Geometry check sheet. Reference: the model listing, model coordinates, mm. A direction names the side the tool comes from. Coordinates: 2 decimals unless noted, no trailing zeros. Loops run counter-clockwise (first coordinate to the right, second up) from the corner with the lowest first, then second, coordinate; pieces in that order, holes last.
Autodesk Inventor part; units mm, degrees
ref_plane "YZ Plane" through (0, 0, 0) normal (1, 0, 0) x (0, 1, 0)
ref_plane "XZ Plane" through (0, 0, 0) normal (0, 1, 0) x (-1, 0, 0)
ref_plane "XY Plane" through (0, 0, 0) normal (0, 0, 1) x (1, 0, 0)
sketch "Sketch1" plane through (0, 0, 0) normal (1, 0, 0) x (0, 1, 0)
  line L0 (0, 0) -> (2400.3, 0)
  line L1 (2400.3, 0) -> (2400.3, -990.6)
  line L2 (2400.3, -990.6) -> (0, -990.6)
  line L3 (0, -990.6) -> (0, 0)
  dimension "d0" = 990.6
  dimension "d1" = 2400.3
extrude "Extrusion1" add sketch "Sketch1" along normal blind 127
sketch "Sketch2" plane through (127, 0, 0) normal (1, 0, 0) x (0, 0, -1)
  line L0 (0, 0) -> (990.6, 0)
  line L1 (927.1, 0) -> (63.5, 0)
  line L2 (63.5, 0) -> (63.5, 2082.8)
  line L3 (63.5, 2082.8) -> (927.1, 2082.8)
  line L4 (927.1, 2082.8) -> (927.1, 0)
  line L5 (990.6, 0) -> (990.6, 2400.3)
  point P0 (63.5, 0)
  point P1 (63.5, 0)
  dimension "d4" = 2082.8
  dimension "d6" = 63.5
  dimension "d7" = 863.6
extrude "Extrusion2" cut sketch "Sketch2" against normal up to surface (127 mm away)
properties part number "Wall_With_Door_For_Attic_Room" material "Wood (Southern Pine)"
1) Mould release check, pull along Z, two halves, no side actions. Record for faces 3 (the flat face through (63, 1217, -990.6)), 4 (the flat face through (64, 1056, -927.1)), 5 (the flat face through (64, 2082.8, -489)), 6 (the flat face through (63, 1183, 0)): +Z half, -Z half, draft (parallel to the pull), parting line (faces both ways), or undercut.
Data:
face 3: -Z half
face 4: undercut
face 5: undercut
face 6: +Z half
2) Section check C-C on z = -740. Record the cut outline in (x, y).
Data:
outline: (0, 2082.8) - (127, 2082.8) - (127, 2400.3) - (0, 2400.3) - close
3) Material ranges on probe 1 along Z at (x, y) = (20, 1375); probe 2 along Y at (x, z) = (117, -202.5), recorded low to high.
Data:
probe 1: z = -990.6 to -927.1, -63.5 to 0
probe 2: y = 2082.8 to 2400.3
4) Section check B-B on x = 40.5. Record the cut outline in (y, z).
Data:
outline: (0, -990.6) - (2400.3, -990.6) - (2400.3, 0) - (0, 0) - (0, -63.5) - (2082.8, -63.5) - (2082.8, -927.1) - (0, -927.1) - close
5) Access from +Z, -Z, +X, -X, +Y, -Y to the whole of each face (thin tool, end or side, straight path). Record for faces 1 (the flat face through (0, 2084, -493)), 2 (the flat face through (64, 1027, -63.5)).
Data:
face 1: +Z, -Z, -X, +Y, -Y
face 2: +X, -X, -Y
6) Section check A-A on y = 173. Record the cut outline in (x, z).
Data:
outline: (0, -990.6) - (127, -990.6) - (127, -927.1) - (0, -927.1) - close; (0, -63.5) - (127, -63.5) - (127, 0) - (0, 0) - close
7) Depth check by flat-ended pin: pin 1 (3 mm diameter, centred on x = 31.5, y = 1318.5, fed in from +Z); pin 2 (8 mm diameter, centred on x = 83, z = -139.5, fed in from -Y). Enter the tip coordinate at first touch or a pass-through.
Data:
pin 1: stops at z = 0
pin 2: stops at y = 2082.8
